Design review of the part built by this model. Coordinates are the model's own, in mm. Coordinates: 2 decimals unless noted, no trailing zeros. Write each loop counter-clockwise with the first axis right and the second up, starting at its lowest first coordinate (ties: lowest second). Pieces come first, ordered by that corner, then holes. Notation, with made-up numbers: (58, 79) -> (110, 79) arc R9 ccw to (110, 83) -> close; hole circle Ø5 at (51.5, 22.5). An arc over 180 degrees is marked (long way). Write item = value, one per line. Start each with the question number.
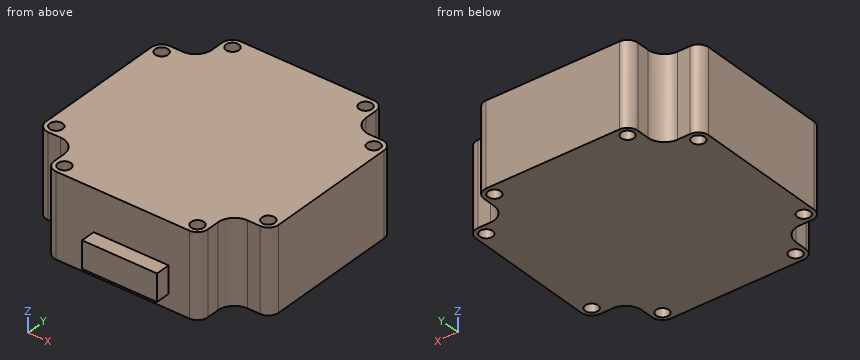
```python
from build123d import *

# Parameters (mm, degrees)
SKETCH_R              = 1.55
PAD_DEPTH             = 20
POLARPATTERN012_COUNT = 4
FILLET004_R           = 4
FILLET005_R           = 2.5
SKETCH019_W           = 18
SKETCH019_H           = 6.5
PAD012_DEPTH          = 31.5


with BuildPart() as part:
    # Sketch → Pad (new body)
    with BuildSketch(Plane.XY):
        Polygon((-28, 0), (-28, 18.5), (-18.5, 18.5), (-18.5, 28), (0, 28), (0, 0), align=None)
        with Locations((-16, 25.5)):
            Circle(SKETCH_R, mode=Mode.SUBTRACT)
        with Locations((-25.5, 16)):
            Circle(SKETCH_R, mode=Mode.SUBTRACT)
    pad = extrude(amount=PAD_DEPTH)

    # PolarPattern012: Pad ×4 about axis
    polarpattern012_axis = Axis((0, 0, 0), (0, 0, 1))
    for i in range(1, POLARPATTERN012_COUNT):
        add(pad.rotate(polarpattern012_axis, i * 360 / POLARPATTERN012_COUNT))

    # Fillet004
    fillet004_edges = [part.edges().sort_by_distance(p)[0] for p in [
        (-18.5, 18.5, 10),
        (18.5, -18.5, 10),
        (-18.5, -18.5, 10),
        (18.5, 18.5, 10),
    ]]
    fillet(fillet004_edges, radius=FILLET004_R)

    # Fillet005
    fillet005_edges = [part.edges().sort_by_distance(p)[0] for p in [
        (-28, -18.5, 10),
        (-18.5, -28, 10),
        (18.5, -28, 10),
        (28, -18.5, 10),
        (28, 18.5, 10),
        (18.5, 28, 10),
        (-18.5, 28, 10),
        (-28, 18.5, 10),
    ]]
    fillet(fillet005_edges, radius=FILLET005_R)

    # Sketch019 → Pad012 (join)
    with BuildSketch(Plane.XZ):
        with Locations((2, 6.75)):
            Rectangle(SKETCH019_W, SKETCH019_H)
    extrude(amount=PAD012_DEPTH)


solid = part.part
```
(1) Take a section at A-A, the plane z = 16.5. Count the separate pieces of the cut face and the enclosed holes in it, then the cut area to 3 significant figures.
(2) For pin 1 Ø10 at (y, z) = (-22, 6.5) entering from +X; pin 2 Ø3.5 at (y, z) = (24.5, 5.5) entering from +X; pin 3 Ø6 at (x, y) = (-3.5, 18.5) entering from -Z; pin 4 Ø1.8 at (x, y) = (2, -29.5) entering from -Z, all flat-tipped, find the tip position at first contact; note any pin that passes through.
(3) For line 1 (Y direction, x = -25.5, z = 11.5); line 2 (Y direction, x = -16, z = 16), list the stretches that pass through material, from the lowest coordinate up.
(4) Take a section at D-D, the plane x = -19.5. State the section outline as (y, z) points, then the cut area to 3 significant figures.
(5) Take a section at B-B, the plane x = -1. State the section outline as (y, z) points.
Report:
q1.separate_pieces = 1
q1.enclosed_holes = 8
q1.area = 2,720 mm2
q2.pin_1 = 27.79
q2.pin_2 = 18.5
q2.pin_3 = 0
q2.pin_4 = 3.5
q3.line_1 = -18.5 to -17.55, -14.45 to 14.45, 17.55 to 18.5
q3.line_2 = -28 to -27.05, -23.95 to 23.95, 27.05 to 28
q4.outline = (-19.85, 0) -> (19.85, 0) -> (19.85, 20) -> (-19.85, 20) -> close
q4.area = 794 mm2
q5.outline = (-31.5, 3.5) -> (-28, 3.5) -> (-28, 0) -> (28, 0) -> (28, 20) -> (-28, 20) -> (-28, 10) -> (-31.5, 10) -> close
